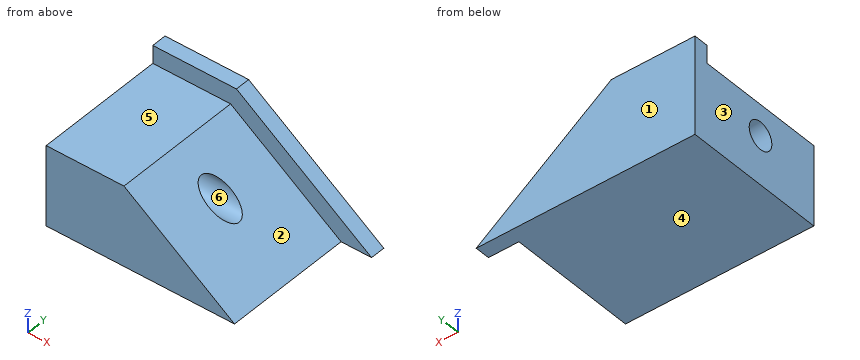
from build123d import *

# Parameters (mm, degrees)
F1_DEPTH = 80.7
F2_DEPTH = 8.3
F3_R     = 7.689637
F4_DEPTH = 105.067501


with BuildPart() as f1:
    # F0 (on Front) → F1 (new body)
    with BuildSketch(Plane.XZ):
        Polygon((-105.066501, 0), (0, 0), (-61.654873, 44.802453), (-105.066501, 44.802453), align=None)
    extrude(amount=F1_DEPTH)

    # F0 (on Front) → F2 (join)
    with BuildSketch(Plane.XZ):
        Polygon((-61.654873, 44.802453), (0, 0), (17.011136, 0), (-58.405232, 54.802453), (-105.066501, 54.802453), (-105.066501, 44.802453), align=None)
    extrude(amount=F2_DEPTH)

    # F3 (on Right) → F4 (cut, through all)
    with BuildSketch(Plane.YZ):
        with Locations((-44.5, 27.401227)):
            Circle(F3_R)
    extrude(amount=-F4_DEPTH, mode=Mode.SUBTRACT)


solid = f1.part
The listing builds one solid part. Answer for the finished solid, in the listing's coordinates (mm). Face numbers are marked on the shaded views. A direction names the side the tool comes from. Coordinates: 2 decimals unless noted, no trailing zeros. Loops run counter-clockwise (first coordinate to the right, second up) from the corner with the lowest first, then second, coordinate; pieces in that order, holes last. Notation, with made-up numbers: (44.5, -31.75) -> (61.5, -31.75) arc R21 ccw to (61.5, -11.75) -> close; hole circle Ø9 at (60, -2.5). An arc over 180 degrees is marked (long way). Answer in a Markdown table with one row per item. Add a question column.
1. Determine the mould class of the marked faces 3, 4, 5 and 6 for opening direction Z: +Z half, -Z half, draft (parallel to the pull), parting line (faces both ways), or undercut.
2. Consider line 1 (Z direction, x = -72, y = -44.5); line 2 (Z direction, x = -51, y = -44.5); line 3 (X direction, y = -41, z = 42). Determine where each line is inside the solid, lowest interval first. Write a range as [from, to].
3. The part is cut by section D-D, the plane y = -5. Write down the section's boundary in (x, z), then the cut area to 3 significant figures.
4. The part is cut by section C-C, the plane x = -56. Write down the section's boundary in (y, z), then the cut area to 3 significant figures.
5. The part is cut by section B-B, the plane z = 24. Write down the section's boundary in (x, y).
6. The part is cut by section A-A, the plane y = -40. Write down the section's boundary in (x, z).
7. Flat-ended cylindrical pins translate along their axes: P1, Ø12, axis at x = -16, y = -56, coming from the +Z side; P2, Ø13, axis at x = -88.5, y = -36.5, coming from the +Z side. Find the tip coordinate at first contact, or state that the pin passes through.
8. For the marked faces 1 and 2, determine the directions among +Z, -Z, +X, -X, +Y, -Y from which every point of the face is accessible in a straight line to the end or side of a thin tool.
Answer below:
| question | item | result |
|---|---|---|
| 1 | face 3 | draft |
| 1 | face 4 | -Z half |
| 1 | face 5 | +Z half |
| 1 | face 6 | undercut |
| 2 | line 1 | [0, 19.71], [35.09, 44.8] |
| 2 | line 2 | [0, 19.71], [35.09, 37.06] |
| 2 | line 3 | [-105.07, -57.8] |
| 3 | outline | (-105.07, 0) -> (17.01, 0) -> (-58.41, 54.8) -> (-105.07, 54.8) -> close |
| 3 | area | 4,620 mm2 |
| 4 | outline | (-80.7, 0) -> (0, 0) -> (0, 53.05) -> (-8.3, 53.05) -> (-8.3, 40.69) -> (-80.7, 40.69) -> close; hole circle Ø15.38 at (-44.5, 27.4) |
| 4 | area | 3,200 mm2 |
| 5 | outline | (-105.07, -80.7) -> (-33.03, -80.7) -> (-33.03, -51.4) -> (-105.07, -51.4) -> close; (-105.07, -37.6) -> (-33.03, -37.6) -> (-33.03, -8.3) -> (-16.02, -8.3) -> (-16.02, 0) -> (-105.07, 0) -> close |
| 6 | outline | (-105.07, 0) -> (0, 0) -> (-29.13, 21.17) -> (-105.07, 21.17) -> close; (-105.07, 33.64) -> (-46.29, 33.64) -> (-61.65, 44.8) -> (-105.07, 44.8) -> close |
| 7 | P1 | z = 15.99 |
| 7 | P2 | z = 44.8 |
| 8 | face 1 | +Z, -Z, +X, -X, +Y |
| 8 | face 2 | +Z, +X, -Y |
